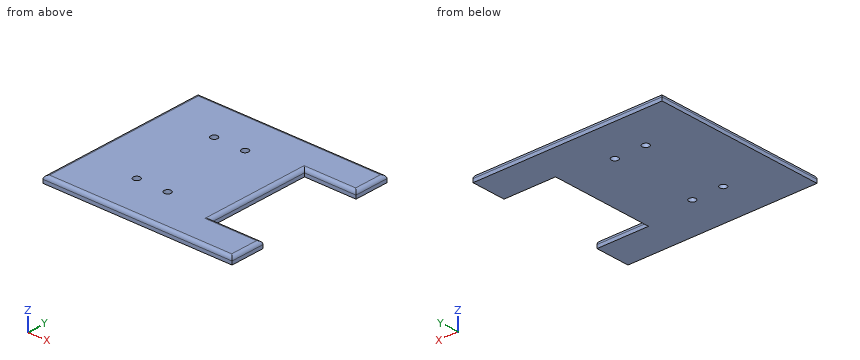
```python
from build123d import *

# Parameters (mm, degrees)
F0_R     = 1
F0_W     = 15
F0_H     = 10
F1_DEPTH = 2
F2_R     = 1


# Not quite as in the source:
# - a feature names something its author has since deleted; it is built from what else it names


with BuildPart() as f1:
    # F0 (on Top) → F1 (new body)
    with BuildSketch(Plane.XY):
        Polygon((-20, -25), (20, -25), (20, -15), (20, 15), (20, 25), (-20, 25), align=None)
        with Locations((-4, -12.5)):
            Circle(F0_R, mode=Mode.SUBTRACT)
        with Locations((5, -12.5)):
            Circle(F0_R, mode=Mode.SUBTRACT)
        with Locations((-4, 12.5)):
            Circle(F0_R, mode=Mode.SUBTRACT)
        with Locations((5, 12.5)):
            Circle(F0_R, mode=Mode.SUBTRACT)
        with Locations((27.5, -20)):
            Rectangle(F0_W, F0_H)
        with Locations((27.5, 20)):
            Rectangle(F0_W, F0_H)
    extrude(amount=-F1_DEPTH)

    # F2
    f2_edges = [f1.edges().sort_by_distance(p)[0] for p in [
        (7.5, 25, 0),
        (-20, 0, 0),
        (35, 20, 0),
        (27.5, 15, 0),
        (20, 0, 0),
        (27.5, -15, 0),
        (35, -20, 0),
        (7.5, -25, 0),
    ]]
    fillet(f2_edges, radius=F2_R)


solid = f1.part
```
Read the model definition and answer for the solid it produces. Units are mm, in the model's axes. Coordinates: 2 decimals unless noted, no trailing zeros. Order: outer loops, then holes, each group sorted by start corner. A loop starts at its lowest first (then second) coordinate and runs counter-clockwise, first axis right, second up. Notation, with made-up numbers: (67.25, 50.25) - (83.25, 50.25) arc R19 ccw to (83.25, 63.25) - close; hole circle Ø3 at (49, 11.25). An arc over 180 degrees is marked (long way). Answer as a JSON object with one key per item and string values. Group by question number.
Item 1: Section C-C (y = -12.5) is taken. Give the vertices of the cut face in (x, z).
Item 2: Section D-D (x = 5) is taken. Give the vertices of the cut face in (y, z).
Item 3: Section B-B (z = -1.6) is taken. Give the vertices of the cut face in (x, y), plus the area to 3 significant figures.
Item 4: Flat-ended cylindrical pins translate along their axes: P1, Ø2.5, axis at x = 5, y = 12.5, coming from the -Z side; P2, Ø0.5, axis at y = -6, z = -1.5, coming from the +X side; P3, Ø1.8, axis at x = 5, y = -12.5, coming from the -Z side. Find the tip coordinate at first contact, or state that the pin passes through.
Item 5: Consider probe 1 along Y at (x, z) = (-4, -0.95); probe 2 along Y at (x, z) = (21.5, -1.8); probe 3 along X at (y, z) = (-12, -1.55). Determine where each line is inside the solid, lowest interval first. Write a range as from..to.
Item 6: Section A-A (x = 29.5) is taken. Give the vertices of the cut face in (y, z).
Results are:
{
 "1": {"outline": "(-20, -2) - (-5, -2) - (-5, 0) - (-19, 0) arc R1 ccw to (-20, -1) - close; (-3, -2) - (4, -2) - (4, 0) - (-3, 0) - close; (6, -2) - (20, -2) - (20, -1) arc R1 ccw to (19, 0) - (6, 0) - close"},
 "2": {"outline": "(-25, -2) - (-13.5, -2) - (-13.5, 0) - (-24, 0) arc R1 ccw to (-25, -1) - close; (-11.5, -2) - (11.5, -2) - (11.5, 0) - (-11.5, 0) - close; (13.5, -2) - (25, -2) - (25, -1) arc R1 ccw to (24, 0) - (13.5, 0) - close"},
 "3": {"outline": "(-20, -25) - (35, -25) - (35, -15) - (20, -15) - (20, 15) - (35, 15) - (35, 25) - (-20, 25) - close; hole circle Ø2 at (-4, -12.5); hole circle Ø2 at (-4, 12.5); hole circle Ø2 at (5, -12.5); hole circle Ø2 at (5, 12.5)", "area": "2,290 mm^2"},
 "4": {"P1": "stops at z = -2", "P2": "stops at x = 20", "P3": "passes through"},
 "5": {"probe 1": "y = -25..-13.5, -11.5..11.5, 13.5..25", "probe 2": "y = -25..-15, 15..25", "probe 3": "x = -20..-4.87, -3.13..4.13, 5.87..20"},
 "6": {"outline": "(-25, -2) - (-15, -2) - (-15, -1) arc R1 ccw to (-16, 0) - (-24, 0) arc R1 ccw to (-25, -1) - close; (15, -2) - (25, -2) - (25, -1) arc R1 ccw to (24, 0) - (16, 0) arc R1 ccw to (15, -1) - close"}
}
